from build123d import *

# Parameters (mm, degrees)
EXTRUDE1_DEPTH             = 4.4
EXTRUDE5_DEPTH             = 6.600446411
EXTRUDE5_DEPTH_BACK        = 6.600446411
EXTRUDE6_REACH             = 8.622
SKETCH15_R                 = 1.35
EXTRUDE6_DIRECTION_2_DEPTH = 1
SKETCH16_R                 = 1.12
EXTRUDE7_DEPTH             = 5


with BuildPart() as part:
    # Sketch1 → Extrude1 (new body)
    with BuildSketch(Plane(origin=(0, 0, 0), x_dir=(1, 0, 0), z_dir=(0, 1, 0))):
        with BuildLine():
            Line((2.076655966, -1.3), (0.642261629, -1.3))
            ThreePointArc((0.642261629, -1.3), (-1.45, 0), (0.642261629, 1.3))
            Line((0.642261629, 1.3), (2.076655966, 1.3))
            ThreePointArc((2.076655966, 1.3), (-2.45, 0), (2.076655966, -1.3))
        make_face()
    extrude(amount=EXTRUDE1_DEPTH)

    # Sketch11 → Extrude5 (cut, two sides)
    with BuildSketch(Plane.XY) as extrude5_sk:
        with BuildLine():
            Line((0.476655966, 4.4), (2.076655966, 4.4))
            Line((2.076655966, 4.4), (2.076655966, 0.7))
            add(Edge.make_bspline(
                [(2.076655966, 0.7), (2.075619632, 1.692222339), (2.074022236, 3.22162422), (0.891869454, 4.093697352), (0.476655966, 4.4)],
                knots=[0, 0, 0, 0, 0.648764953, 1, 1, 1, 1], degree=3))
        make_face()
    extrude(amount=EXTRUDE5_DEPTH, mode=Mode.SUBTRACT)
    extrude(extrude5_sk.sketch, amount=-EXTRUDE5_DEPTH_BACK, mode=Mode.SUBTRACT)

    # Sketch15 → Extrude6 (add, up to next)
    with BuildSketch(Plane(origin=(-3.143655548, 1.144197046, 0), x_dir=(0, 0, -1), z_dir=(0.9396926207859126, -0.34202014332565683, 0)), mode=Mode.PRIVATE) as extrude6_sk1:
        with Locations(Location((0, 2.028113142, 0), (0, 0, 90))):
            Circle(SKETCH15_R)
    extrude6_tool1 = extrude(extrude6_sk1.sketch, amount=EXTRUDE6_REACH, mode=Mode.PRIVATE) - part.part
    add(extrude6_tool1.solids().sort_by_distance((-2.45, 3.05, 0))[0])

    # Sketch15 → Extrude6 direction 2 (add)
    with BuildSketch(Plane(origin=(-3.143655548, 1.144197046, 0), x_dir=(0, 0, -1), z_dir=(0.9396926207859126, -0.34202014332565683, 0))):
        with Locations(Location((0, 2.028113142, 0), (0, 0, 90))):
            Circle(SKETCH15_R)
    extrude(amount=-EXTRUDE6_DIRECTION_2_DEPTH)

    # Sketch16 → Extrude7 (add)
    with BuildSketch(Plane(origin=(-4.083348168, 1.486217189, 0), x_dir=(0, 0, 1), z_dir=(-0.9396926207859126, 0.34202014332565694, 0))):
        with Locations(Location((0, 2.028113142, 0), (0, 0, 90))):
            Circle(SKETCH16_R)
    extrude(amount=EXTRUDE7_DEPTH)


solid = part.part
For this review, take the finished solid that the model builds, in its own axes (mm). A direction names the side the tool comes from. Round coordinates to 2 decimals unless told otherwise and drop trailing zeros. Loops run counter-clockwise (first coordinate to the right, second up) from the corner with the lowest first, then second, coordinate; pieces in that order, holes last. Notation, with made-up numbers: (-19, -26) - (37, -26) arc R11 ccw to (37, -7) - close; hole circle Ø2 at (-39.5, 63). An arc over 180 degrees is marked (long way). One line per question, with ' | ' between items.
Q1. Take a section at A-A (x = 0). Give the boundary of the cut face in (y, z).
Taken from the geometry:
outline: (0, -2.45) - (4.4, -2.45) - (4.4, -1.45) - (0, -1.45) - close; (0, 1.45) - (4.4, 1.45) - (4.4, 2.45) - (0, 2.45) - close
Q2. Take a section at B-B (z = 0). Give the boundary of the cut face in (x, y).
Taken from the geometry:
outline: (-8.47, 4.05) - (-3.77, 2.34) - (-3.85, 2.12) - (-2.45, 1.61) - (-2.45, 0) - (-1.45, 0) - (-1.45, 4.4) - (-2.21, 4.4) - (-2.93, 4.66) - (-3.01, 4.44) - (-7.71, 6.15) - close
Q3. Tool access review of faces 1 (the cylindrical face through (-1.45, 2.17, 0.04)), 2 (the flat face through (1, 2, -1.3)): name each direction out of +Z, -Z, +X, -X, +Y, -Y from which nothing blocks a thin tool from reaching the whole face with its end or side.
Taken from the geometry:
face 1: +Y, -Y | face 2: +X, +Y, -Y
Q4. For line 1 along Z through (x, y) = (0, 2.55); line 2 along Z through (x, y) = (1, 3.5); line 3 along Y through (x, z) = (-1.75, -1.15), list the stretches that pass through material, from the lowest coordinate up. Write a range as [from, to].
Taken from the geometry:
line 1: z = [-2.45, -1.45], [1.45, 2.45] | line 2: z = [-2.24, -1.3], [1.3, 2.24] | line 3: y = [0, 4.4]
Q5. For pin 1 (1.5 mm diameter, centred on y = 2.5, z = 1, fed in from +X); pin 2 (2.5 mm diameter, centred on x = -1.5, z = -0.5, fed in from +Y); pin 3 (1.6 mm diameter, centred on x = 1, y = 1, fed in from +Z), all flat-tipped, find the tip position at first contact; note any pin that passes through.
Taken from the geometry:
pin 1: stops at x = 2.05 | pin 2: stops at y = 4.57 | pin 3: stops at z = 2.44
